Print and shaded views of the part. All mm, measured from the part's lowest x, y and z. Coordinates: 2 decimals unless noted, no trailing zeros. Order: outer loops, then holes, each group sorted by start corner. A loop starts at its lowest first (then second) coordinate and runs counter-clockwise, first axis right, second up. Notation, with made-up numbers: M 24.25,25 L 47.25,25 A22 cw 47.25,32 Z; hole C 19.25,7.25 d5. An arc over 180 degrees is marked long. One line per item, written item: value.
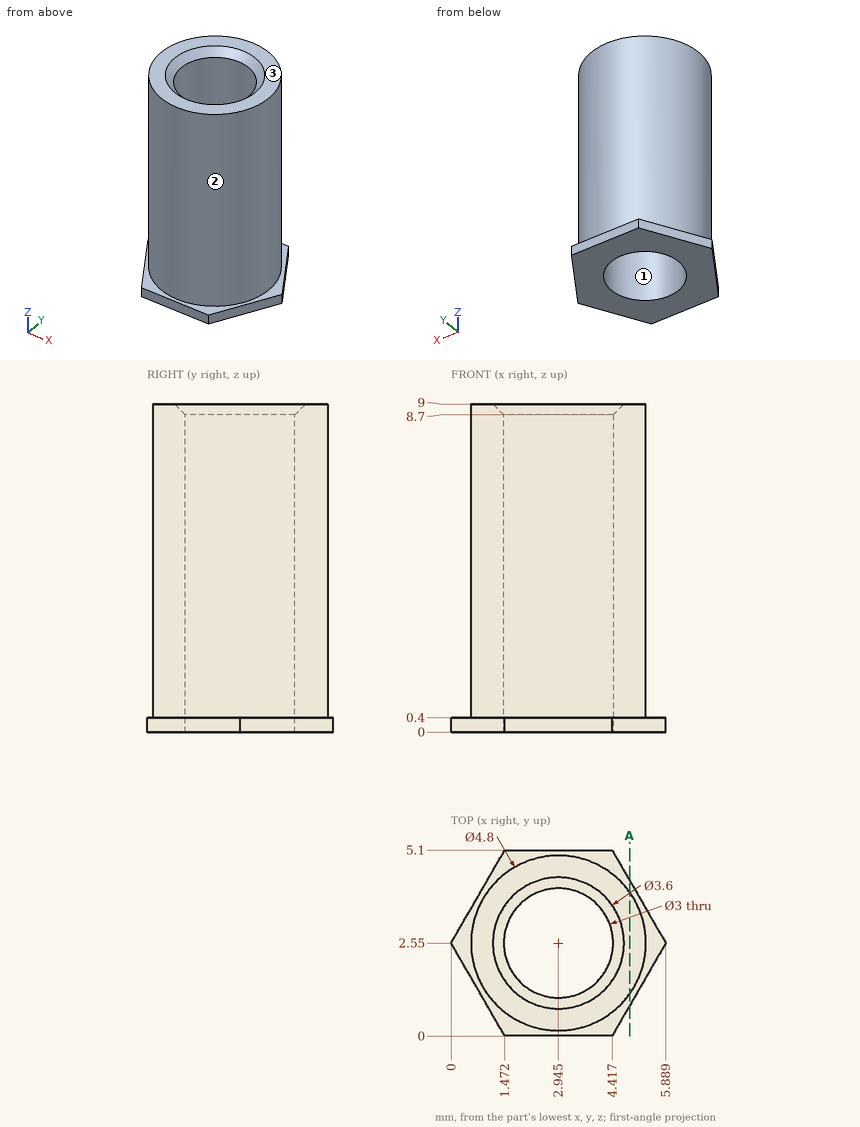
Q1. Drill centre lines: line 1 along Y through (x, z) = (2.9, 8); line 2 along Y through (x, z) = (2.1, 4.25) (1 decimal); line 3 along X through (y, z) = (2.9, 5.5) (1 decimal). Where is each one in solid material? Low to high.
Recorded:
line 1: y = 0.15 to 1.05, 4.05 to 4.95
line 2: y = 0.3 to 1.3, 3.8 to 4.8
line 3: x = 0.6 to 1.5, 4.4 to 5.3
Q2. Mould opens along X. For the marked faces 1, 2 and 3 say: released by +X, released by -X, zero draft, split by the parting line, or undercut.
Recorded:
face 1: undercut
face 2: split by the parting line
face 3: zero draft
Q3. Slice it at A-A (x = 4.9). List the corners of the cut face in (y, z).
Recorded:
outline: M 0.84,0 L 4.26,0 L 4.26,0.4 L 3.94,0.4 L 3.94,9 L 1.16,9 L 1.16,0.4 L 0.84,0.4 Z
Q4. Pin check, flat tip, straight feed: pin 1 Ø2 at (y, z) = (4, 4) entering from +X. Stop position of the tip, or through.
Recorded:
pin 1: stops at x = 5.3
